from build123d import *

# Parameters (mm, degrees)
SKETCH_1_W                  = 120
SKETCH_1_H                  = 42
EXTRUDE_1_DEPTH             = 2
SKETCH_2_W                  = 106
SKETCH_2_H                  = 42
EXTRUDE_2_DEPTH             = 14.5
HOLE_WIZARD_M3_1_AT_2_COUNT = 2
HOLE_WIZARD_M3_1_AT_2_PITCH = 17.5


with BuildPart() as part:
    # ｽｹｯﾁ1 → ﾎﾞｽ - 押し出し1 (new body)
    with BuildSketch(Plane(origin=(0, 0, 0), x_dir=(1, 0, 0), z_dir=(0, 1, 0))):
        Rectangle(SKETCH_1_W, SKETCH_1_H)
    extrude(amount=EXTRUDE_1_DEPTH)

    # ｽｹｯﾁ2 → ﾎﾞｽ - 押し出し2 (add)
    with BuildSketch(Plane(origin=(0, 2, 0), x_dir=(1, 0, 0), z_dir=(0, 1, 0))):
        Rectangle(SKETCH_2_W, SKETCH_2_H)
    extrude(amount=EXTRUDE_2_DEPTH)

    # ｽｹｯﾁ4 → M3 すきま穴1 (revolve, cut)
    with BuildSketch(Plane(origin=(-57, 2, -17.5), x_dir=(0, 0, 1), z_dir=(1, 0, 0))):
        Polygon((0, 0), (0, 6.081549114), (1.8, 5), (1.8, 0), align=None)
    hole_wizard_m3_1 = revolve(axis=Axis((-57, 8.35, -17.5), (0, -1, 0)), mode=Mode.SUBTRACT)

    # M3 すきま穴1 at 2: M3 すきま穴1 ×2
    with Locations(*[(0, 0, i * HOLE_WIZARD_M3_1_AT_2_PITCH) for i in range(1, HOLE_WIZARD_M3_1_AT_2_COUNT)]):
        add(hole_wizard_m3_1, mode=Mode.SUBTRACT)

    # ﾐﾗｰ1: M3 すきま穴1 across plane
    add(hole_wizard_m3_1.mirror(Plane.XY), mode=Mode.SUBTRACT)

    # ﾐﾗｰ1 copy 1 sketch → ﾐﾗｰ1 copy 1 (revolve, cut)
    with BuildSketch(Plane(origin=(-57, 2, 0), x_dir=(0, 0, -1), z_dir=(1, 0, 0))):
        Polygon((0, 0), (0, -6.081549114), (1.8, -5), (1.8, 0), align=None)
    revolve(axis=Axis((-57, 8.35, 0), (0, 1, 0)), mode=Mode.SUBTRACT)

    # ﾐﾗｰ2: M3 すきま穴1 across plane
    add(hole_wizard_m3_1.mirror(Plane(origin=(0, 0, 0), x_dir=(0, 0, 1), z_dir=(1, 0, 0))), mode=Mode.SUBTRACT)

    # ﾐﾗｰ2 copy 1 sketch → ﾐﾗｰ2 copy 1 (revolve, cut)
    with BuildSketch(Plane(origin=(57, 2, 0), x_dir=(0, 0, 1), z_dir=(-1, 0, 0))):
        Polygon((0, 0), (0, -6.081549114), (1.8, -5), (1.8, 0), align=None)
    revolve(axis=Axis((57, 8.35, 0), (0, 1, 0)), mode=Mode.SUBTRACT)

    # ﾐﾗｰ2 copy 2 sketch → ﾐﾗｰ2 copy 2 (revolve, cut)
    with BuildSketch(Plane(origin=(57, 2, 17.5), x_dir=(0, 0, -1), z_dir=(-1, 0, 0))):
        Polygon((0, 0), (0, 6.081549114), (1.8, 5), (1.8, 0), align=None)
    revolve(axis=Axis((57, 8.35, 17.5), (0, -1, 0)), mode=Mode.SUBTRACT)

    # ﾐﾗｰ2 copy 3 sketch → ﾐﾗｰ2 copy 3 (revolve, cut)
    with BuildSketch(Plane(origin=(57, 2, 0), x_dir=(0, 0, -1), z_dir=(-1, 0, 0))):
        Polygon((0, 0), (0, 6.081549114), (1.8, 5), (1.8, 0), align=None)
    revolve(axis=Axis((57, 8.35, 0), (0, -1, 0)), mode=Mode.SUBTRACT)


solid = part.part
Work out the finished part from the listing and answer in its coordinate system (mm). A direction names the side the tool comes from. Round coordinates to 2 decimals unless told otherwise and drop trailing zeros. Write each loop counter-clockwise with the first axis right and the second up, starting at its lowest first coordinate (ties: lowest second). Pieces come first, ordered by that corner, then holes.
1) A tool of negligible diameter and unlimited length cuts with its end or side. For faces 4 (the flat face through (60, 1, 0)), 5 (the flat face through (55, 2, 0)), 6 (the flat face through (-55, 2, 0)), from which of +Z, -Z, +X, -X, +Y, -Y can it reach the whole face along a straight path? Write none if from no direction.
2) A cutting plane is placed at D-D (y = 11.5). Give the vertices of the cut face in (x, z).
3) A cutting plane is placed at C-C (z = -3). Give the vertices of the cut face in (x, y).
4) A cutting plane is placed at B-B (x = 57). Give the vertices of the cut face in (y, z), plus the area to 3 significant figures.
5) Straight lines are drawn through the part: line 1 (X direction, y = 1.6, z = 0); line 2 (Z direction, x = -57, y = 1.25); line 3 (X direction, y = 12.5, z = -7). For each, find the intervals that lie inside material, in ascending order.
6) A cutting plane is placed at A-A (z = 17.5). Give the vertices of the cut face in (x, y), plus the area to 3 significant figures.
7) The mould has two halves that part along Z. Classify faces 1 (the flat face through (-53, 9, 0)), 2 (the cylindrical face through (55.243, 1.014, -0.39)), 3 (the flat face through (-1, 8, -21)): pulls with the +Z half, pulls with the -Z half, needs draft (parallel to the pull), parting line crosses it, or undercut.
8) Given pin 1 Ø8 at (y, z) = (12.5, 13) entering from -X; pin 2 Ø4.5 at (x, z) = (57, 17.5) entering from -Y; pin 3 Ø7 at (y, z) = (8, 0.5) entering from +X; pin 4 Ø7.5 at (x, z) = (58, 9.5) entering from +Y, each flat-ended and moving along its own axis, determine where each tip first touches the part or whether it passes through.
Completed:
1. face 4: +Z, -Z, +X, +Y, -Y
1. face 5: +Z, -Z, +X, +Y
1. face 6: +Z, -Z, -X, +Y
2. outline: (-53, -21) - (53, -21) - (53, 21) - (-53, 21) - close
3. outline: (-60, 0) - (60, 0) - (60, 2) - (53, 2) - (53, 16.5) - (-53, 16.5) - (-53, 2) - (-60, 2) - close
4. outline: (0, -21) - (2, -21) - (2, -19.3) - (0, -19.3) - close; (0, -15.7) - (2, -15.7) - (2, -1.8) - (0, -1.8) - close; (0, 1.8) - (2, 1.8) - (2, 15.7) - (0, 15.7) - close; (0, 19.3) - (2, 19.3) - (2, 21) - (0, 21) - close
4. area: 62.4 mm2
5. line 1: x = -60 to -58.8, -55.2 to 55.2, 58.8 to 60
5. line 2: z = -21 to -19.3, -15.7 to -1.8, 1.8 to 15.7, 19.3 to 21
5. line 3: x = -53 to 53
6. outline: (-60, 0) - (-58.8, 0) - (-58.8, 2) - (-60, 2) - close; (-55.2, 0) - (55.2, 0) - (55.2, 2) - (53, 2) - (53, 16.5) - (-53, 16.5) - (-53, 2) - (-55.2, 2) - close; (58.8, 0) - (60, 0) - (60, 2) - (58.8, 2) - close
6. area: 1,760 mm2
7. face 1: needs draft
7. face 2: undercut
7. face 3: pulls with the -Z half
8. pin 1: stops at x = -53
8. pin 2: stops at y = 0
8. pin 3: stops at x = 53
8. pin 4: stops at y = 2
